Input: part model. Units: mm. Frame: model coordinates. Face numbers are marked on the shaded views. A direction names the side the tool comes from. Coordinates: 2 decimals unless noted, no trailing zeros. Order: outer loops, then holes, each group sorted by start corner. A loop starts at its lowest first (then second) coordinate and runs counter-clockwise, first axis right, second up.
from build123d import *

# Parameters (mm, degrees)
SKETCH1_W           = 10.16
SKETCH1_H           = 10.16
BOSS_EXTRUDE1_DEPTH = 81.915
SKETCH10_R          = 2.6035
CUT_EXTRUDE6_DEPTH  = 82.915
SKETCH11_R          = 3.7465
CUT_EXTRUDE7_DEPTH  = 1.27
SKETCH12_W          = 12.065
SKETCH12_H          = 3.175
BOSS_EXTRUDE4_DEPTH = 11.303
SKETCH13_W          = 12.065
SKETCH13_H          = 3.175
BOSS_EXTRUDE5_DEPTH = 11.303


with BuildPart() as part:
    # Sketch1 → Boss-Extrude1 (new body)
    with BuildSketch(Plane(origin=(0, 0, 0), x_dir=(0, 0, -1), z_dir=(1, 0, 0))):
        with Locations((5.08, 5.08)):
            Rectangle(SKETCH1_W, SKETCH1_H)
    extrude(amount=BOSS_EXTRUDE1_DEPTH)

    # Sketch10 → Cut-Extrude6 (cut, through all)
    with BuildSketch(Plane(origin=(81.915, 0, 0), x_dir=(0, 0, -1), z_dir=(1, 0, 0))):
        with Locations((5.08, 5.08)):
            Circle(SKETCH10_R)
    extrude(amount=-CUT_EXTRUDE6_DEPTH, mode=Mode.SUBTRACT)

    # Sketch11 → Cut-Extrude7 (cut)
    with BuildSketch(Plane.XY):
        with Locations((40.9575, 5.08)):
            Circle(SKETCH11_R)
    extrude(amount=-CUT_EXTRUDE7_DEPTH, mode=Mode.SUBTRACT)

    # Sketch12 → Boss-Extrude4 (add)
    with BuildSketch(Plane.XZ):
        with Locations((40.9575, -1.5875)):
            Rectangle(SKETCH12_W, SKETCH12_H)
    extrude(amount=BOSS_EXTRUDE4_DEPTH)

    # Sketch13 → Boss-Extrude5 (add)
    with BuildSketch(Plane(origin=(0, 10.16, 0), x_dir=(1, 0, 0), z_dir=(0, 1, 0))):
        with Locations((40.9575, 1.5875)):
            Rectangle(SKETCH13_W, SKETCH13_H)
    extrude(amount=BOSS_EXTRUDE5_DEPTH)


solid = part.part
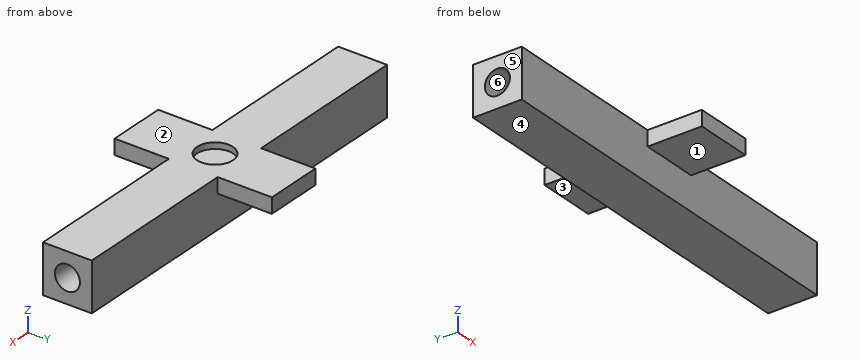
Item 1: Access query for the marked faces 1, 2 and 3. Directions: +Z, -Z, +X, -X, +Y, -Y. A direction counts if a zero-diameter tool reaches every point of the face in a straight line with its end or side. Return the directions, or none.
Response values:
face 1: -Z, +X, -X, -Y
face 2: +Z, +X, -X, +Y, -Y
face 3: -Z, +X, -X, +Y
Item 2: Cut plane B-B on z = -5.08. Return loops of the section in (x, y) (1 decimal), then the cut area to 3 significant figures.
Response values:
outline: (0, 0) - (81.9, 0) - (81.9, 2.5) - (0, 2.5) - close; (0, 7.7) - (81.9, 7.7) - (81.9, 10.2) - (0, 10.2) - close
area: 406 mm2
Item 3: Draft query along Z for the marked faces 4, 5 and 6. Return one class per face: pulls with the +Z half, pulls with the -Z half, needs draft (parallel to the pull), parting line crosses it, or undercut.
Response values:
face 4: pulls with the -Z half
face 5: needs draft
face 6: undercut
Item 4: Cut plane D-D on y = -7. Return loops of the section in (x, z) (3 decimals).
Response values:
outline: (34.925, -3.175) - (46.99, -3.175) - (46.99, 0) - (34.925, 0) - close
Item 5: Pin query (flat end, axial travel): pin 1 Ø2.5 at (y, z) = (17.5, -1.5) entering from -X (3 decimals); pin 2 Ø3 at (x, z) = (58.5, -4.5) entering from +Y; pin 3 Ø1 at (y, z) = (17, -2) entering from +X. Return the tip coordinate at first contact, or that it passes through.
Response values:
pin 1: stops at x = 34.925
pin 2: stops at y = 10.16
pin 3: stops at x = 46.99
Item 6: Cut plane C-C on x = 59. Return loops of the section in (y, z).
Response values:
outline: (0, -10.16) - (10.16, -10.16) - (10.16, 0) - (0, 0) - close; hole circle Ø5.21 at (5.08, -5.08)
Item 7: Ray query, probe 1 along Y at (x, z) = (20, -5.08); probe 2 along X at (y, z) = (-8, -2.5) (3 decimals); probe 3 along Y at (x, z) = (28, -1.5). Return the intervals inside material, ascending.
Response values:
probe 1: y = 0 to 2.48, 7.68 to 10.16
probe 2: x = 34.925 to 46.99
probe 3: y = 0 to 10.16
Item 8: Cut plane A-A on y = 5.08. Return loops of the section in (x, z) (1 decimal), then the cut area to 3 significant figures.
Response values:
outline: (0, -10.2) - (81.9, -10.2) - (81.9, -7.7) - (0, -7.7) - close; (0, -2.5) - (81.9, -2.5) - (81.9, 0) - (44.7, 0) - (44.7, -1.3) - (37.2, -1.3) - (37.2, 0) - (0, 0) - close
area: 396 mm2
